Check sheet for the drawn part. Datum: minimum x, y, z corner. Units: mm. A direction names the side the tool comes from. Coordinates: 2 decimals unless noted, no trailing zeros. Loops run counter-clockwise (first coordinate to the right, second up) from the corner with the lowest first, then second, coordinate; pieces in that order, holes last.
Q1. Sectioned sample at C-C (y = 6.75). Enter the section's corners in (x, z).
Q2. Access from +Z, -Z, +X, -X, +Y, -Y to the whole of each face (thin tool, end or side, straight path). Record for the marked faces 1, 2 and 3.
Q3. Material ranges on probe 1 along X at (y, z) = (11.25, 3.75) (1 decimal); probe 2 along Z at (x, y) = (3.75, 2.75); probe 3 along Y at (x, z) = (4.75, 3.5), recorded low to high.
Q4. Sectioned sample at A-A (x = 3.8). Enter the section's corners in (y, z).
Q5. Go/stop test with flat-tipped pins: P1, Ø1.5, axis at y = 2.5, z = 2.5, coming from the -X side; P2, Ø3, axis at y = 1.5, z = 4.5, coming from the +X side; P3, Ø4, axis at y = 5.5, z = 2.5, coming from the -X side. Record where each tip stops, or that it passes through.
Q6. Mould release check, pull along Z, two halves, no side actions. Record for the marked faces 4, 5, 6 and 7: +Z half, -Z half, draft (parallel to the pull), parting line (faces both ways), or undercut.
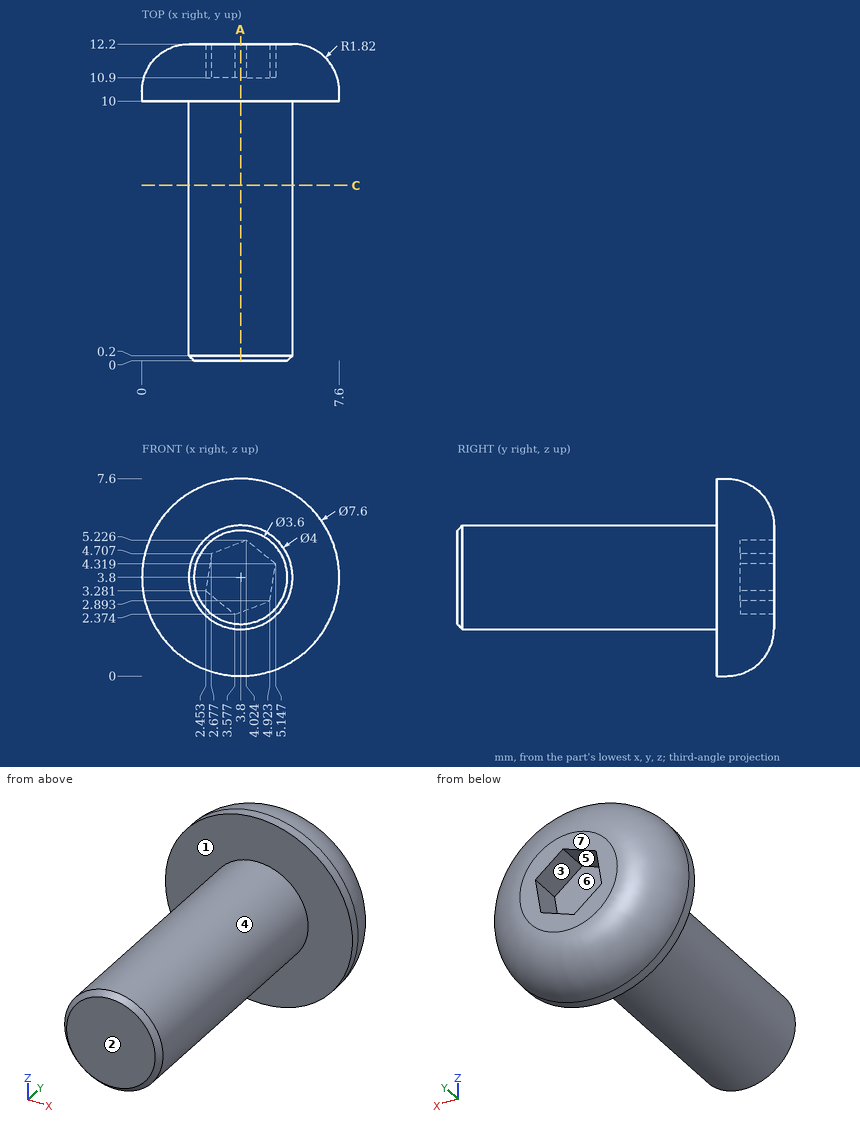
Geometry check:
1. outline: circle Ø4 at (3.8, 3.8)
2. face 1: -Y
2. face 2: +Z, -Z, +X, -X, -Y
2. face 3: +Y
3. probe 1: x = 0.2 to 2.5, 5.1 to 7.4
3. probe 2: z = 1.8 to 5.8
3. probe 3: y = 0 to 10.9
4. outline: (0, 2) - (0.2, 1.8) - (10, 1.8) - (10, 0) - (10.38, 0) arc R1.82 ccw to (12.2, 1.82) - (12.2, 2.46) - (10.9, 2.46) - (10.9, 5.14) - (12.2, 5.14) - (12.2, 5.78) arc R1.82 ccw to (10.38, 7.6) - (10, 7.6) - (10, 5.8) - (0.2, 5.8) - (0, 5.6) - close
5. P1: stops at x = 1.88
5. P2: stops at x = 5.8
5. P3: stops at x = 1.8
6. face 4: parting line
6. face 5: undercut
6. face 6: undercut
6. face 7: draft
